Geometry check sheet. Reference: the model listing, model coordinates, mm. A direction names the side the tool comes from. Give positions to 0.01 mm unless a question says otherwise; leave off trailing zeros. Order: outer loops, then holes, each group sorted by start corner. A loop starts at its lowest first (then second) coordinate and runs counter-clockwise, first axis right, second up. Notation, with made-up numbers: M 74,83 L 78,83 A13 cw 78,99 Z; hole C 45.5,29 d1. An arc over 180 degrees is marked long. Use CSV: the item, a comma, the result in double quotes. Start each with the question number.
from build123d import *

# Parameters (mm, degrees)
SKETCH1_W           = 24.5
SKETCH1_H           = 32
SKETCH1_R           = 1.05
BOSS_EXTRUDE1_DEPTH = 3
SKETCH3_W           = 24.5
SKETCH3_H           = 3
BOSS_EXTRUDE3_DEPTH = 17.48
SKETCH4_R           = 1
CUT_EXTRUDE1_DEPTH  = 10


with BuildPart() as part:
    # Sketch1 → Boss-Extrude1 (new body)
    with BuildSketch(Plane(origin=(0, 0, 0), x_dir=(1, 0, 0), z_dir=(0, 1, 0))):
        Rectangle(SKETCH1_W, SKETCH1_H)
        with Locations(Location((8, 6, 0), (0, 0, 270))):
            Circle(SKETCH1_R, mode=Mode.SUBTRACT)
        with Locations(Location((-8, 6, 0), (0, 0, 270))):
            Circle(SKETCH1_R, mode=Mode.SUBTRACT)
    extrude(amount=BOSS_EXTRUDE1_DEPTH)

    # Sketch3 → Boss-Extrude3 (add)
    with BuildSketch(Plane(origin=(0, 3, 0), x_dir=(1, 0, 0), z_dir=(0, 1, 0))):
        with Locations((0, -14.5)):
            Rectangle(SKETCH3_W, SKETCH3_H)
    extrude(amount=BOSS_EXTRUDE3_DEPTH)

    # Sketch4 → Cut-Extrude1 (cut)
    with BuildSketch(Plane(origin=(0, 0, 13), x_dir=(-1, 0, 0), z_dir=(0, 0, -1))):
        with Locations((8, 11.74)):
            Circle(SKETCH4_R)
        with Locations((-8, 11.74)):
            Circle(SKETCH4_R)
    extrude(amount=-CUT_EXTRUDE1_DEPTH, mode=Mode.SUBTRACT)


solid = part.part
(1) Sectioned sample at A-A on x = -8. Record the cut outline in (y, z), then the cut area to 3 significant figures.
(2) Sectioned sample at D-D on x = 0.5. Record the cut outline in (y, z), then the cut area to 3 significant figures.
(3) Access from +Z, -Z, +X, -X, +Y, -Y to the whole of each face (thin tool, end or side, straight path). Record for faces 4 (the face through (0, 12, 13)), 5 (the face through (0, 0, 0)).
(4) Draft check along Y on faces 1 (the face through (0, 3, -2)), 2 (the face through (-12.25, 2, 6)), 3 (the face through (8.217, 10.764, 14.479)). Enter one of: +Y half, -Y half, draft (parallel to the pull), parting line (faces both ways), or undercut.
(5) Thickness scan on line 1 (Y direction, x = 8, z = 14.7); line 2 (X direction, y = 1.85, z = -6); line 3 (Y direction, x = -1.25, z = -5). Record the ranges inside material, lowest first.
(6) Sectioned sample at C-C on y = 11.74. Record the cut outline in (x, z), then the cut area to 3 significant figures.
(7) Sectioned sample at B-B on z = -6. Record the cut outline in (x, y), then the cut area to 3 significant figures.
(8) Go/stop test with flat-tipped pins: P1, Ø2.5, axis at x = -8, y = 11.74, coming from the -Z side; P2, Ø2.5, axis at x = -8, z = -6, coming from the +Y side. Record where each tip stops, or that it passes through.
Responses:
1,outline,"M 0,-16 L 3,-16 L 3,-7.05 L 0,-7.05 Z; M 0,-4.95 L 3,-4.95 L 3,13 L 10.74,13 L 10.74,16 L 0,16 Z; M 12.74,13 L 20.48,13 L 20.48,16 L 12.74,16 Z"
1,area,"136 mm2"
2,outline,"M 0,-16 L 3,-16 L 3,13 L 20.48,13 L 20.48,16 L 0,16 Z"
2,area,"148 mm2"
3,face 4,"-Z, +X, -X, +Y"
3,face 5,"+Z, -Z, +X, -X, -Y"
4,face 1,"+Y half"
4,face 2,"draft"
4,face 3,"undercut"
5,line 1,"0 to 10.74, 12.74 to 20.48"
5,line 2,"-12.25 to -9.05, -6.95 to 6.95, 9.05 to 12.25"
5,line 3,"0 to 3"
6,outline,"M -12.25,13 L -9,13 L -9,16 L -12.25,16 Z; M -7,13 L 7,13 L 7,16 L -7,16 Z; M 9,13 L 12.25,13 L 12.25,16 L 9,16 Z"
6,area,"61.5 mm2"
7,outline,"M -12.25,0 L -9.05,0 L -9.05,3 L -12.25,3 Z; M -6.95,0 L 6.95,0 L 6.95,3 L -6.95,3 Z; M 9.05,0 L 12.25,0 L 12.25,3 L 9.05,3 Z"
7,area,"60.9 mm2"
8,P1,"z = 13"
8,P2,"y = 3"
